Check sheet for the modelled part. Datum: model origin and axes. Units: mm. Face numbers are marked on the shaded views. A direction names the side the tool comes from. Coordinates: 2 decimals unless noted, no trailing zeros. Write each loop counter-clockwise with the first axis right and the second up, starting at its lowest first coordinate (ties: lowest second). Pieces come first, ordered by that corner, then holes. Notation, with made-up numbers: (44, 4.5) -> (94, 4.5) arc R25 cw to (94, 29.5) -> close; hole circle Ø8 at (-37, 59.5). An arc over 180 degrees is marked (long way). Put each result on its own line as item: value.
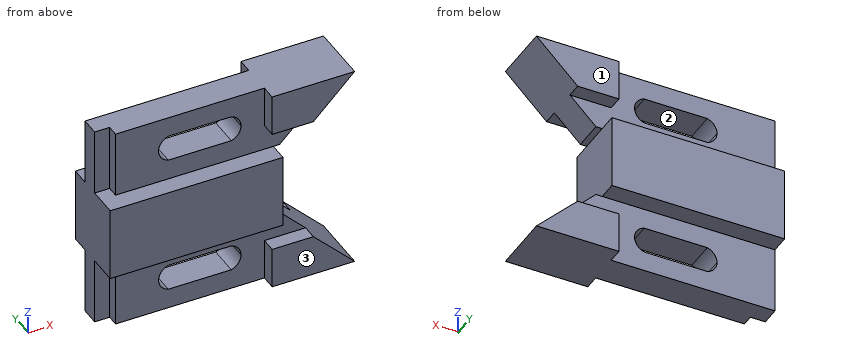
```python
from build123d import *

# Parameters (mm, degrees)
F0_W      = 31.242
F0_H      = 12.7
F1_DEPTH  = 28.575
F0_W_2    = 69.596
F0_H_2    = 6.35
F2_DEPTH  = 15.875
F4_DEPTH  = 26.925
F6_DEPTH  = 20.575
F9_DEPTH  = 6.35
F10_DEPTH = 6.35


with BuildPart() as f1:
    # F0 (on Top) → F1 (new body)
    with BuildSketch(Plane.XY):
        with Locations((89.027, 6.35)):
            Rectangle(F0_W, F0_H)
        with Locations((89.027, -6.35)):
            Rectangle(F0_W, F0_H)
        Polygon((73.406, 0), (0, 0), (0, -1.524), (6.35, -1.524), (6.35, -6.35), (69.596, -6.35), (69.596, -12.7), (73.406, -12.7), align=None)
        Polygon((0, 6.35), (0, 0), (73.406, 0), (73.406, 12.7), (69.596, 12.7), (69.596, 6.35), align=None)
    extrude(amount=F1_DEPTH)

    # F0 (on Top) → F2 (join)
    with BuildSketch(Plane.XY):
        with Locations((34.798, 9.525)):
            Rectangle(F0_W_2, F0_H_2)
        Polygon((0, 6.35), (0, 0), (73.406, 0), (73.406, 12.7), (69.596, 12.7), (69.596, 6.35), align=None)
        Polygon((73.406, 0), (0, 0), (0, -1.524), (6.35, -1.524), (6.35, -6.35), (69.596, -6.35), (69.596, -12.7), (73.406, -12.7), align=None)
        Polygon((6.35, -1.524), (0, -1.524), (0, -6.35), (0, -12.7), (69.596, -12.7), (69.596, -6.35), (6.35, -6.35), align=None)
        Polygon((73.406, -14.224), (73.406, -12.7), (69.596, -12.7), (0, -12.7), (0, -14.224), align=None)
        Polygon((69.596, 12.7), (73.406, 12.7), (73.406, 14.224), (0, 14.224), (0, 12.7), align=None)
    extrude(amount=-F2_DEPTH)

    # F3 (on face) → F4 (cut, through all)
    with BuildSketch(Plane.XZ.offset(12.7)):
        Polygon((104.648, 0), (104.648, 28.575), (76.073, 0), align=None)
    extrude(amount=-F4_DEPTH, mode=Mode.SUBTRACT)

    # F5 (on face) → F6 (cut, through all)
    with BuildSketch(Plane.XZ.offset(6.35)):
        with BuildLine():
            ThreePointArc((28.7761162011, 19.939), (25.7851595792, 17.8276992138), (24.638, 14.351))
            Line((24.638, 14.351), (30.48, 14.351))
            Line((30.48, 14.351), (36.322, 14.351))
            ThreePointArc((36.322, 14.351), (35.1748404208, 17.8276992138), (32.1838837989, 19.939))
            Line((32.1838837989, 19.939), (28.7761162011, 19.939))
        make_face()
        with BuildLine():
            Line((30.48, 14.351), (24.638, 14.351))
            ThreePointArc((24.638, 14.351), (25.7851595792, 10.8743007862), (28.7761162011, 8.763))
            Line((28.7761162011, 8.763), (32.1838837989, 8.763))
            ThreePointArc((32.1838837989, 8.763), (35.1748404208, 10.8743007862), (36.322, 14.351))
            Line((36.322, 14.351), (30.48, 14.351))
        make_face()
        with BuildLine():
            ThreePointArc((32.1838837989, 19.939), (35.1748404208, 17.8276992138), (36.322, 14.351))
            Line((36.322, 14.351), (48.006, 14.351))
            ThreePointArc((48.006, 14.351), (49.1531595792, 17.8276992138), (52.1441162011, 19.939))
            Line((52.1441162011, 19.939), (32.1838837989, 19.939))
        make_face()
        with BuildLine():
            ThreePointArc((52.1441162011, 19.939), (49.1531595792, 17.8276992138), (48.006, 14.351))
            Line((48.006, 14.351), (53.848, 14.351))
            Line((53.848, 14.351), (59.69, 14.351))
            ThreePointArc((59.69, 14.351), (58.5428404208, 17.8276992138), (55.5518837989, 19.939))
            Line((55.5518837989, 19.939), (52.1441162011, 19.939))
        make_face()
        with BuildLine():
            Line((53.848, 14.351), (48.006, 14.351))
            ThreePointArc((48.006, 14.351), (49.1531595792, 10.8743007862), (52.1441162011, 8.763))
            Line((52.1441162011, 8.763), (55.5518837989, 8.763))
            ThreePointArc((55.5518837989, 8.763), (58.5428404208, 10.8743007862), (59.69, 14.351))
            Line((59.69, 14.351), (53.848, 14.351))
        make_face()
        with BuildLine():
            Line((48.006, 14.351), (36.322, 14.351))
            ThreePointArc((36.322, 14.351), (35.1748404208, 10.8743007862), (32.1838837989, 8.763))
            Line((32.1838837989, 8.763), (52.1441162011, 8.763))
            ThreePointArc((52.1441162011, 8.763), (49.1531595792, 10.8743007862), (48.006, 14.351))
        make_face()
    extrude(amount=-F6_DEPTH, mode=Mode.SUBTRACT)

    # F8 (on face) → F9 (cut)
    with BuildSketch(Plane(origin=(0, 12.7, 0), x_dir=(-1, 0, 0), z_dir=(0, 1, 0))):
        Polygon((-69.596, 0), (-69.596, 11.049), (-87.122, 11.049), (-76.073, 0), (-73.406, 0), align=None)
    extrude(amount=-F9_DEPTH, mode=Mode.SUBTRACT)

    # F7 (on face) → F10 (cut)
    with BuildSketch(Plane.XZ.offset(12.7)):
        Polygon((87.122, 11.049), (69.596, 11.049), (69.596, 0), (73.406, 0), (76.073, 0), align=None)
    extrude(amount=-F10_DEPTH, mode=Mode.SUBTRACT)

    # F11: F1 across face


with BuildPart() as f1_1:
    add(f1.part)
    add(f1.part.mirror(Plane(origin=(36.703, 0, -15.875), x_dir=(1, 0, 0), z_dir=(0, 0, -1))))


solid = f1_1.part
```
Q1. Depth check by flat-ended pin: P1, Ø5.5, axis at x = 79, z = 18.5, coming from the +Y side; P2, Ø8, axis at y = 2.5, z = -19, coming from the +X side; P3, Ø4, axis at y = -4.5, z = -46.5, coming from the -X side. Enter the tip coordinate at first touch or a pass-through.
Recorded:
P1: stops at y = 12.7
P2: stops at x = 73.41
P3: stops at x = 6.35
Q2. Material ranges on line 1 along Z through (x, y) = (72.5, 9.5) (3 decimals); line 2 along Z through (x, y) = (38, -5) (3 decimals); line 3 along X through (y, z) = (-10.25, -28), recorded low to high.
Recorded:
line 1: z = -60.325 to -42.799, -31.75 to 0, 11.049 to 28.575
line 2: z = -60.325 to -51.689, -40.513 to 8.763, 19.939 to 28.575
line 3: x = 0 to 73.41
Q3. Tool access check on the marked faces 1, 2 and 3. Record the directions out of +Z, -Z, +X, -X, +Y, -Y that give a thin tool (end or side, any length) a straight path to the whole face; none if there is none.
Recorded:
face 1: +Z, +X, -X, +Y
face 2: +Y, -Y
face 3: -Z, +X, -X, -Y
Q4. Cross-section at A-A (y = 7.5). Record the cut outline in (x, z) (3 decimals).
Recorded:
outline: (0, -31.75) -> (73.406, -31.75) -> (73.406, 0) -> (0, 0) -> close; (69.596, -60.325) -> (104.648, -60.325) -> (87.122, -42.799) -> (69.596, -42.799) -> close; (69.596, 11.049) -> (87.122, 11.049) -> (104.648, 28.575) -> (69.596, 28.575) -> close
Q5. Cross-section at D-D (z = -49). Record the cut outline in (x, y).
Recorded:
outline: (0, -1.52) -> (6.35, -1.52) -> (6.35, -6.35) -> (25.41, -6.35) -> (25.41, 6.35) -> (0, 6.35) -> close; (58.92, -6.35) -> (69.6, -6.35) -> (69.6, -12.7) -> (93.32, -12.7) -> (93.32, 12.7) -> (69.6, 12.7) -> (69.6, 6.35) -> (58.92, 6.35) -> close
Q6. Cross-section at B-B (x = 48.5). Record the cut outline in (y, z) (3 decimals).
Recorded:
outline: (-14.224, -31.75) -> (-6.35, -31.75) -> (-6.35, -40.513) -> (6.35, -40.513) -> (6.35, -31.75) -> (14.224, -31.75) -> (14.224, 0) -> (6.35, 0) -> (6.35, 8.763) -> (-6.35, 8.763) -> (-6.35, 0) -> (-14.224, 0) -> close; (-6.35, -60.325) -> (6.35, -60.325) -> (6.35, -51.689) -> (-6.35, -51.689) -> close; (-6.35, 19.939) -> (6.35, 19.939) -> (6.35, 28.575) -> (-6.35, 28.575) -> close
Q7. Cross-section at C-C (x = 10). Record the cut outline in (y, z) (3 decimals), plus the area to 3 significant figures.
Recorded:
outline: (-14.224, -31.75) -> (-6.35, -31.75) -> (-6.35, -60.325) -> (6.35, -60.325) -> (6.35, -31.75) -> (14.224, -31.75) -> (14.224, 0) -> (6.35, 0) -> (6.35, 28.575) -> (-6.35, 28.575) -> (-6.35, 0) -> (-14.224, 0) -> close
area: 1,630 mm2
